The model under review builds one solid part; all positions refer to its coordinate system, in mm. A direction names the side the tool comes from. Coordinates: 2 decimals unless noted, no trailing zeros. Order: outer loops, then holes, each group sorted by start corner. A loop starts at its lowest first (then second) coordinate and runs counter-clockwise, first axis right, second up.
from build123d import *

# Parameters (mm, degrees)
F1_DEPTH  = 190.5
F2_W      = 190.5
F2_H      = 79.375
F3_DEPTH  = 3.175
F4_W      = 149.86
F4_H      = 79.375
F5_DEPTH  = 19.05
F6_W      = 139.7
F6_H      = 12.7
F7_DEPTH  = 127
F8_R      = 2.38125
F9_DEPTH  = 12.7
F10_R     = 2.38125
F11_DEPTH = 25.4
F12_W     = 20.32
F12_H     = 12.7
F13_DEPTH = 19.05
F14_W     = 20.32
F14_H     = 12.7
F15_DEPTH = 19.05
F17_DEPTH = 203.2
F18_W     = 13.97
F18_H     = 61.595
F19_DEPTH = 254
F20_W     = 180.34
F20_H     = 45.9946300644
F21_DEPTH = 5.08


with BuildPart() as f1:
    # F0 (on Right) → F1 (new body)
    with BuildSketch(Plane.YZ):
        with BuildLine():
            Line((-76.2, 0), (0, 0))
            Line((0, 0), (0, 79.375))
            ThreePointArc((0, 79.375), (-26.424895677, 28.4793998499), (-76.2, 0))
        make_face()
    extrude(amount=F1_DEPTH)

    # F2 (on face) → F3 (join)
    with BuildSketch(Plane(origin=(0, 0, 0), x_dir=(-1, 0, 0), z_dir=(0, 1, 0))):
        with Locations((-95.25, 39.6875)):
            Rectangle(F2_W, F2_H)
    extrude(amount=F3_DEPTH)

    # F4 (on face) → F5 (join)
    with BuildSketch(Plane(origin=(0, 3.175, 0), x_dir=(-1, 0, 0), z_dir=(0, 1, 0))):
        with Locations((-95.25, 39.6875)):
            Rectangle(F4_W, F4_H)
    extrude(amount=F5_DEPTH)

    # F6 (on face) → F7 (cut)
    with BuildSketch(Plane.XY.offset(79.375)):
        with Locations((95.25, 12.7)):
            Rectangle(F6_W, F6_H)
    extrude(amount=-F7_DEPTH, mode=Mode.SUBTRACT)

    # F8 (on face) → F9 (cut)
    with BuildSketch(Plane(origin=(0, 22.225, 0), x_dir=(-1, 0, 0), z_dir=(0, 1, 0))):
        with Locations((-132.08, 50.8)):
            Circle(F8_R)
        with BuildLine():
            ThreePointArc((-56.03875, 50.8), (-58.42, 53.18125), (-60.80125, 50.8))
            ThreePointArc((-60.80125, 50.8), (-58.42, 48.41875), (-56.03875, 50.8))
        make_face()
    extrude(amount=-F9_DEPTH, mode=Mode.SUBTRACT)

    # F10 (on face) → F11 (cut)
    with BuildSketch(Plane(origin=(0, 0, 0), x_dir=(1, 0, 0), z_dir=(0, 0, -1))):
        with BuildLine():
            ThreePointArc((154.78125, 63.5), (152.4, 65.88125), (150.01875, 63.5))
            ThreePointArc((150.01875, 63.5), (152.4, 61.11875), (154.78125, 63.5))
        make_face()
        with Locations((38.1, 63.5)):
            Circle(F10_R)
    extrude(amount=-F11_DEPTH, mode=Mode.SUBTRACT)

    # F12 (on face) → F13 (join)
    with BuildSketch(Plane(origin=(0, 3.175, 0), x_dir=(-1, 0, 0), z_dir=(0, 1, 0))):
        with Locations((-180.34, 73.025)):
            Rectangle(F12_W, F12_H)
    extrude(amount=F13_DEPTH)

    # F14 (on face) → F15 (join)
    with BuildSketch(Plane(origin=(0, 3.175, 0), x_dir=(-1, 0, 0), z_dir=(0, 1, 0))):
        with Locations((-10.16, 73.025)):
            Rectangle(F14_W, F14_H)
    extrude(amount=F15_DEPTH)

    # F16 (on face) → F17 (cut)
    with BuildSketch(Plane.YZ.offset(190.5)):
        with BuildLine():
            ThreePointArc((-1.905, 53.34), (-21.8614303996, 25.0364303996), (-50.165, 5.08))
            Line((-50.165, 5.08), (-1.905, 5.08))
            Line((-1.905, 5.08), (-1.905, 53.34))
        make_face()
    extrude(amount=-F17_DEPTH, mode=Mode.SUBTRACT)

    # F18 (on face) → F19 (cut)
    with BuildSketch(Plane.YZ.offset(170.18)):
        with Locations((10.16, 35.8775)):
            Rectangle(F18_W, F18_H)
    extrude(amount=-F19_DEPTH, mode=Mode.SUBTRACT)

    # F20 (on face) → F21 (cut)
    with BuildSketch(Plane(origin=(0, 0, 0), x_dir=(1, 0, 0), z_dir=(0, 0, -1))):
        with Locations((95.25, 24.9023150322)):
            Rectangle(F20_W, F20_H)
    extrude(amount=-F21_DEPTH, mode=Mode.SUBTRACT)


solid = f1.part
(1) Insertion check: pin 1 Ø4.5 at (x, z) = (132.08, 50.8) entering from -Y; pin 2 Ø8 at (x, y) = (90.5, -54.5) entering from +Z; pin 3 Ø1 at (x, y) = (47.5, -64) entering from +Z. Each pin has a flat end and moves straight along its axis. Give the tip position at first contact, or say it passes through.
(2) The part is to be moulded in two halves that separate along Y. For faces 1 (the face through (96, -49, 5.08)), 2 (the face through (97, 22.225, 40)), 3 (the face through (97, 6, 79.375)), say which applies: +Y half, -Y half, draft (parallel to the pull), parting line (faces both ways), or undercut.
(3) Consider section A-A (x = 33.5). Give the boundary of the cut face in (y, z) (3 decimals).
(4) Consider section B-B (y = -46). Give the boundary of the cut face in (x, z).
(5) Consider section C-C (x = 58.42). Give the boundary of the cut face in (y, z) (3 decimals), then the cut area to 3 significant figures.
(6) Tool access review of faces 4 (the face through (170.18, 18, 28)), 5 (the face through (185.42, -25, 3)), 6 (the face through (23, 17.145, 35)): name each direction out of +Z, -Z, +X, -X, +Y, -Y from which nothing blocks a thin tool from reaching the whole face with its end or side.
(7) Consider section D-D (z = 63). Give the boundary of the cut face in (x, y) (3 decimals).
(8) Wall thickness on line 1 (X direction, y = -63.5, z = 1.3); line 2 (Y direction, x = 36, z = 41) (3 decimals); line 3 (Z direction, x = 58, y = 21) (3 decimals): over which ranges is each line inside the solid? List them lowest first.
Findings:
1. pin 1: stops at y = -11.44
1. pin 2: stops at z = 9.96
1. pin 3: stops at z = 3.92
2. face 1: undercut
2. face 2: +Y half
2. face 3: draft
3. outline: (-76.2, 0) - (-47.9, 0) - (-47.9, 5.08) - (-50.165, 5.08) arc R101.6 ccw to (-1.905, 53.34) - (-1.905, 0) - (6.35, 0) - (6.35, 5.08) - (3.175, 5.08) - (3.175, 66.675) - (6.35, 66.675) - (6.35, 79.375) - (0, 79.375) arc R101.6 cw to start; (19.05, 0) - (22.225, 0) - (22.225, 79.375) - (19.05, 79.375) - close
4. outline: (0, 0) - (5.08, 0) - (5.08, 5.08) - (0, 5.08) - close; (0, 7.17) - (190.5, 7.17) - (190.5, 12.6) - (0, 12.6) - close; (185.42, 0) - (190.5, 0) - (190.5, 5.08) - (185.42, 5.08) - close
5. outline: (-76.2, 0) - (-47.9, 0) - (-47.9, 5.08) - (-50.165, 5.08) arc R101.6 ccw to (-1.905, 53.34) - (-1.905, 0) - (6.35, 0) - (6.35, 5.08) - (3.175, 5.08) - (3.175, 66.675) - (6.35, 66.675) - (6.35, 79.375) - (0, 79.375) arc R101.6 cw to start; (19.05, 0) - (22.225, 0) - (22.225, 48.419) - (19.05, 48.419) - close; (19.05, 53.181) - (22.225, 53.181) - (22.225, 79.375) - (19.05, 79.375) - close
5. area: 1,230 mm2
6. face 4: -Z, +X, +Y
6. face 5: -Z
6. face 6: +X, -X
7. outline: (0, -4.649) - (190.5, -4.649) - (190.5, 3.175) - (0, 3.175) - close; (20.32, 17.145) - (25.4, 17.145) - (25.4, 19.05) - (165.1, 19.05) - (165.1, 17.145) - (170.18, 17.145) - (170.18, 22.225) - (20.32, 22.225) - close
8. line 1: x = 0 to 35.72, 40.48 to 150.02, 154.78 to 190.5
8. line 2: y = -16.189 to -8.85, -1.905 to 3.175, 19.05 to 22.225
8. line 3: z = 0 to 48.456, 53.144 to 79.375
